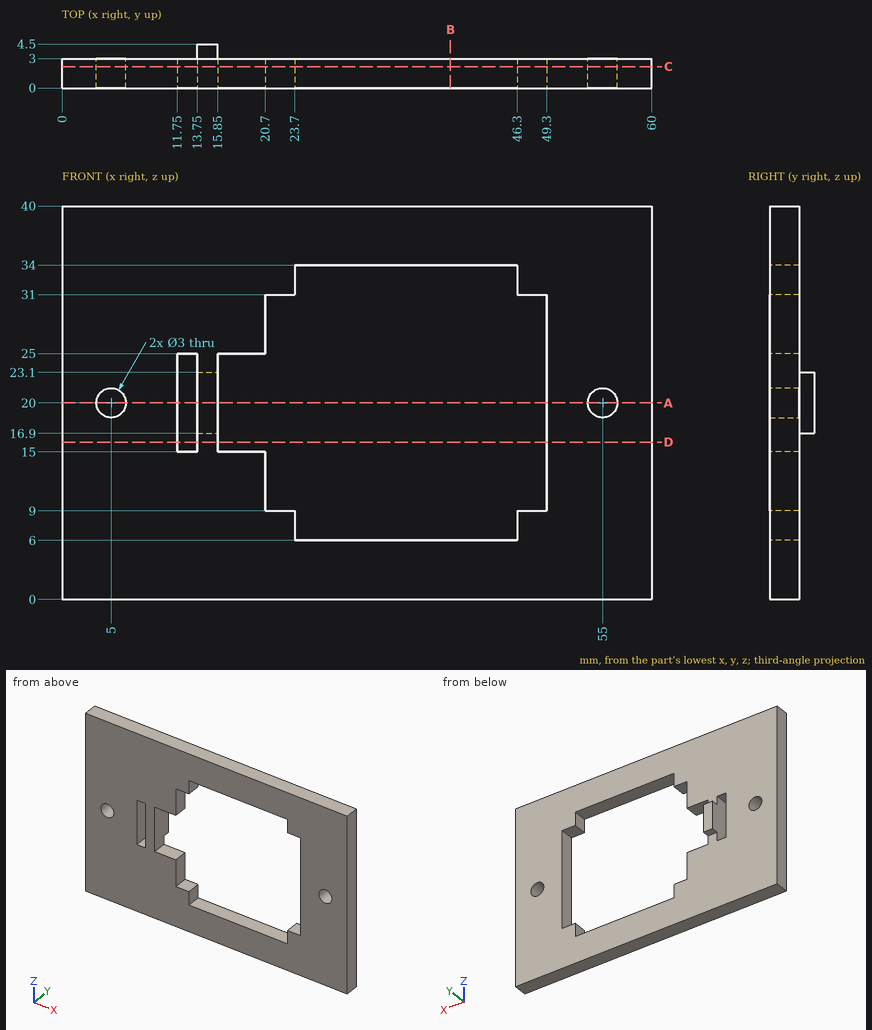
Could you check a few things on this drawing? It's one solid part, dimensions in mm from its lowest x, y, z. Give positions to 0.01 mm unless a question says otherwise; leave off trailing zeros. Loops run counter-clockwise (first coordinate to the right, second up) from the corner with the lowest first, then second, coordinate; pieces in that order, holes last. Notation, with made-up numbers: M -11,0 L -3,0 A26 ccw -3,23 Z; hole C 59,51.5 d8. An arc over 180 degrees is marked long. Return JSON: item names as keys, results as strings.
Item 1: Imagine slicing it at B-B on x = 39.5. List the corners of the cut face in (y, z) for me, then the cut area to 3 significant figures.
A:
{"outline": "M 0,0 L 3,0 L 3,6 L 0,6 Z; M 0,34 L 3,34 L 3,40 L 0,40 Z", "area": "36.0 mm^2"}
Item 2: Imagine slicing it at A-A on z = 20. List the corners of the cut face in (x, y) for me.
A:
{"outline": "M 0,0 L 3.5,0 L 3.5,3 L 0,3 Z; M 6.5,0 L 11.75,0 L 11.75,3 L 6.5,3 Z; M 13.75,0 L 15.85,0 L 15.85,4.5 L 13.75,4.5 Z; M 49.3,0 L 53.5,0 L 53.5,3 L 49.3,3 Z; M 56.5,0 L 60,0 L 60,3 L 56.5,3 Z"}
Item 3: Imagine slicing it at D-D on z = 16. List the corners of the cut face in (x, y) for me, then the cut area to 4 significant figures.
A:
{"outline": "M 0,0 L 11.75,0 L 11.75,3 L 0,3 Z; M 13.75,0 L 15.85,0 L 15.85,3 L 13.75,3 Z; M 49.3,0 L 60,0 L 60,3 L 49.3,3 Z", "area": "73.65 mm^2"}
Item 4: I'm going to push flat-ended pins straight in: pin 1 Ø1.5 at (y, z) = (1.5, 6) entering from -X; pin 2 Ø8 at (x, z) = (42, 15) entering from +Y. Where does each tip first touch, or does it pass through?
A:
{"pin 1": "stops at x = 0", "pin 2": "passes through"}
Item 5: Imagine slicing it at C-C on y = 2.2. List the corners of the cut face in (x, z) for me.
A:
{"outline": "M 0,0 L 60,0 L 60,40 L 0,40 Z; hole C 5,20 d3; hole M 11.75,15 L 13.75,15 L 13.75,25 L 11.75,25 Z; hole M 15.85,15 L 20.7,15 L 20.7,9 L 23.7,9 L 23.7,6 L 46.3,6 L 46.3,9 L 49.3,9 L 49.3,31 L 46.3,31 L 46.3,34 L 23.7,34 L 23.7,31 L 20.7,31 L 20.7,25 L 15.85,25 Z; hole C 55,20 d3"}
Item 6: Please list where these lines run through material, in increasing order: line 1 (X direction, y = 0.95, z = 17.5); line 2 (X direction, y = 0.9, z = 20); line 3 (Z direction, x = 47.5, y = 0.8).
A:
{"line 1": "x = 0 to 11.75, 13.75 to 15.85, 49.3 to 60", "line 2": "x = 0 to 3.5, 6.5 to 11.75, 13.75 to 15.85, 49.3 to 53.5, 56.5 to 60", "line 3": "z = 0 to 9, 31 to 40"}
